The model under review builds one solid part; all positions refer to its coordinate system, in mm. Give positions to 0.01 mm unless a question says otherwise; leave off trailing zeros. Loops run counter-clockwise (first coordinate to the right, second up) from the corner with the lowest first, then second, coordinate; pieces in that order, holes last. Notation, with made-up numbers: (3.5, -13) - (46.5, -13) arc R37 cw to (46.5, 26) - close; hole circle Ø8 at (61, 1). An arc over 180 degrees is marked (long way). Answer as a JSON object with one key per item and string values.
from build123d import *

# Parameters (mm, degrees)
SKETCH1_R           = 17
SKETCH1_R_2         = 13
BOSS_EXTRUDE1_DEPTH = 124.5
CUT_EXTRUDE2_START  = 10
CUT_EXTRUDE2_DEPTH  = 50
THREAD1_PITCH       = 3
CHAMFER2_SIZE       = 1


with BuildPart() as part:
    # Sketch1 → Boss-Extrude1 (new, symmetric)
    with BuildSketch(Plane(origin=(0, 0, 0), x_dir=(1, 0, 0), z_dir=(0, 1, 0))):
        with Locations(Location((0, 0, 0), (0, 0, 270))):
            Circle(SKETCH1_R)
        with Locations(Location((0, 0, 0), (0, 0, 270))):
            Circle(SKETCH1_R_2, mode=Mode.SUBTRACT)
    extrude(amount=BOSS_EXTRUDE1_DEPTH, both=True)

    # Sketch3 → Cut-Extrude2 (cut)
    with BuildSketch(Plane(origin=(0, 87, 0), x_dir=(1, 0, 0), z_dir=(0, 1, 0)).offset(CUT_EXTRUDE2_START)):
        with BuildLine():
            Line((0, 0), (14.722431864, 8.5))
            ThreePointArc((14.722431864, 8.5), (0, 17), (-14.722431864, 8.5))
            Line((-14.722431864, 8.5), (0, 0))
        make_face()
    extrude(amount=-CUT_EXTRUDE2_DEPTH, mode=Mode.SUBTRACT)

    # Thread1: the profile of Thread Profile1 profile screwed along a left-hand helix of 4 turns, 10 arcs to a turn; built about Z, then put on its axis
    thread1_z = Axis((0, 0, 0), (0, 0, 1))
    thread1_corners = [(17.0003, 0, -0.000173205), (17.0003, 0, 2.625173197), (15.376202375, 0, 1.687499996), (15.376202375, 0, 0.937499996)]
    with BuildLine(mode=Mode.PRIVATE) as thread1_profile:
        Line(thread1_corners[0], thread1_corners[1])
        Line(thread1_corners[1], thread1_corners[2])
        Line(thread1_corners[2], thread1_corners[3])
        Line(thread1_corners[3], thread1_corners[0])
    thread1_cap = Face(thread1_profile.wire())
    thread1_turn_angles = [0, -18, -36, -54, -72, -90, -108, -126, -144, -162, -180, -198, -216, -234, -252, -270, -288, -306, -324, -342, -360]
    thread1_turn_weights = [1, 0.9510565162951535, 1, 0.9510565162951535, 1, 0.9510565162951535, 1, 0.9510565162951535, 1, 0.9510565162951535, 1, 0.9510565162951535, 1, 0.9510565162951535, 1, 0.9510565162951535, 1, 0.9510565162951535, 1, 0.9510565162951535, 1]
    thread1_turn_rails = [Edge.make_bspline([Vector(p[0], p[1], 0).rotate(thread1_z, thread1_turn_angles[k]) / thread1_turn_weights[k] + Vector(0, 0, p[2] + -THREAD1_PITCH * thread1_turn_angles[k] / 360) for k in range(21)], [0, 0, 0, 1, 1, 2, 2, 3, 3, 4, 4, 5, 5, 6, 6, 7, 7, 8, 8, 9, 9, 10, 10, 10], 2, thread1_turn_weights) for p in thread1_corners]
    thread1_turn_sides = [Face.make_surface_from_curves(thread1_turn_rails[p[0]], thread1_turn_rails[p[1]]) for p in [(0, 1), (1, 2), (2, 3), (3, 0)]]
    thread1 = Plane(origin=(0, -125.5, 0), x_dir=(1, 0, 0), z_dir=(0, 1, 0)) * Solid(Shell([*[p.moved(Location((0, 0, THREAD1_PITCH * i))) for i in range(4) for p in thread1_turn_sides], thread1_cap, thread1_cap.rotate(thread1_z, -1440).moved(Location((0, 0, -THREAD1_PITCH * -1440 / 360)))]))
    add(thread1, mode=Mode.SUBTRACT)

    # Chamfer2
    chamfer2_edges = [part.edges().sort_by_distance(p)[0] for p in [
        (-8.48872702, -124.5, -14.728934571),
    ]]
    chamfer(chamfer2_edges, length=CHAMFER2_SIZE)


solid = part.part
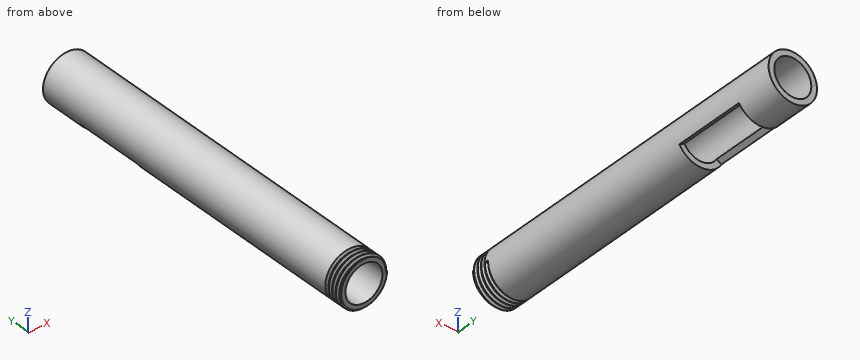
Q1. To check wall thickness, follow probe 1 along Y at (x, z) = (-3.5, 15.5); probe 2 along X at (y, z) = (72, 0); probe 3 along Y at (x, z) = (4.5, -14). State the ranges of each line that lie inside material, in increasing order. Write a range as [from, to].
Results:
{"probe 1": "y = [-124.5, -124], [-122.66, -121], [-119.66, -118], [-116.66, -115], [-113.66, 124.5]", "probe 2": "x = [-17, -13], [13, 17]", "probe 3": "y = [-124.5, 47], [97, 124.5]"}
Q2. Clearance check with flat-ended pins moving along their axes: pin 1 Ø12 at (x, y) = (-6.5, 94) entering from -Z; pin 2 Ø8 at (y, z) = (0, -1.5) entering from -X; pin 3 Ø2 at (x, y) = (9.5, -33.5) entering from +Z; pin 4 Ø1.5 at (x, y) = (-2, -29.5) entering from +Z. State where each tip first meets the part, or that it passes through.
Results:
{"pin 1": "stops at z = -16.95", "pin 2": "stops at x = -17", "pin 3": "stops at z = 14.72", "pin 4": "stops at z = 16.95"}
Q3. Consider section B-B, the plane x = 0. State how many separate pieces and enclosed holes the cut face has, plus the area to 3 significant figures.
Results:
{"separate pieces": "3", "enclosed holes": "0", "area": "1,770 mm^2"}
Q4. Consider section A-A, the plane y = 16.5. State the section outline as (x, z) points, plus the area to 3 significant figures.
Results:
{"outline": "circle Ø34 at (0, 0); hole circle Ø26 at (0, 0)", "area": "377 mm^2"}
